For this review, take the finished solid that the model builds, in its own axes (mm). A direction names the side the tool comes from. Coordinates: 2 decimals unless noted, no trailing zeros. Order: outer loops, then holes, each group sorted by start corner. A loop starts at its lowest first (then second) coordinate and runs counter-clockwise, first axis right, second up. Notation, with made-up numbers: M 25.25,-7.75 L 84.25,-7.75 A27 cw 84.25,15.25 Z; hole C 63.5,52 d2. An arc over 180 degrees is marked long. Use CSV: the item, a comma, the result in double quotes.
Autodesk Inventor part; units mm, degrees
ref_plane "Start Plane" through (0, 0, 50.831) normal (0, 0, 1) x (1, 0, 0)
ref_plane "End Plane" through (0, 0, 1320.8) normal (0, 0, 1) x (1, 0, 0)
ref_plane "Work Plane4" through (-2540, 0, 50.831) normal (0, 0, -1) x (-1, 0, 0)
ref_plane "Start Plane" through (0, 0, 50.831) normal (0, 0, 1) x (1, 0, 0)
ref_plane "End Plane" through (0, 0, 1320.8) normal (0, 0, 1) x (1, 0, 0)
sketch "Sketch" plane through (0, 0, 0) normal (0, 0, 1) x (1, 0, 0)
  line L0 (-25.4, -31.75) -> (-25.4, 31.75)
  line L1 (-19.05, 38.1) -> (19.05, 38.1)
  line L2 (25.4, 31.75) -> (25.4, -31.75)
  line L3 (19.05, -38.1) -> (-19.05, -38.1)
  arc A0 (-25.4, -31.75) -> (-19.05, -38.1) centre (-19.05, -31.75) ccw
  arc A1 (-19.05, 38.1) -> (-25.4, 31.75) centre (-19.05, 31.75) ccw
  arc A2 (25.4, 31.75) -> (19.05, 38.1) centre (19.05, 31.75) ccw
  arc A3 (19.05, -38.1) -> (25.4, -31.75) centre (19.05, -31.75) ccw
  arc A4 (-19.05, 34.925) -> (-22.225, 31.75) centre (-19.05, 31.75) ccw
  line L4 (-19.05, 34.925) -> (19.05, 34.925)
  arc A5 (22.225, 31.75) -> (19.05, 34.925) centre (19.05, 31.75) ccw
  line L5 (22.225, 31.75) -> (22.225, -31.75)
  arc A6 (19.05, -34.925) -> (22.225, -31.75) centre (19.05, -31.75) ccw
  line L6 (19.05, -34.925) -> (-19.05, -34.925)
  arc A7 (-22.225, -31.75) -> (-19.05, -34.925) centre (-19.05, -31.75) ccw
  line L7 (-22.225, -31.75) -> (-22.225, 31.75)
  line L8 (0, 55.1812) -> (0, -55.1812) construction
  line L9 (-37.4012, 0) -> (37.4012, 0) construction
  dimension "d10" = 76.2
  dimension "d11" = 50.8
  dimension "d12" = 3.175
  dimension "d15" = 38.1
  dimension "d16" = 25.4
  dimension "d17" = 6.35
extrude "Body" add sketch "Sketch" along normal up to surface (1269.969 mm away) from surface at 50.831
sketch "Sketch3" plane through (0, 0, 0) normal (0, 0, 1) x (1, 0, 0)
  line L0 (0, 0) -> (10, 0)
ref_plane "Work Plane3" through (0, 0, 0) normal (0, -1, 0) x (1, 0, 0)
ref_plane "Work Plane4" through (-2540, 0, 50.831) normal (0, 0, -1) x (-1, 0, 0)
split "Split1" plane through (-2540, 0, 50.831) removes the side toward (0, 0, -1)
sketch "Sketch4" plane through (0, 0, 0) normal (0, -1, 0) x (1, 0, 0)
  line L0 (-2, 50.831) -> (12, 50.831)
  line L1 (-2, 1320.8) -> (12, 1320.8)
  dimension "d19" = 1269.969
equation "\"d10\" = G_H"
equation "\"d11\" = G_W"
equation "\"d12\" = G_T"
equation "\"d15\" = 0.5 * d10"
equation "\"d16\" = 0.5 * d11"
equation "\"d17\" = G_IR"
equation "\"d3\" = G_L"
equation "\"G_W\" = 50.8"
equation "\"G_H\" = 76.2"
equation "\"G_T\" = 3.175"
equation "\"G_IR\" = 6.35"
equation "\"G_L\" = d19"
equation "\"G_OFFSET_START\" = -50.831"
equation "\"G_OFFSET_END\" = 0"
equation "\"d13\" = -G_OFFSET_START"
equation "\"d14\" = G_OFFSET_END + B_L"
equation "\"B_L\" = 1320.8"
properties part number "AISC - 3 x 2 x 1/8 - 49.999" material "Steel, Mild"
Item 1: For faces 5 (the face through (0, -38.1, 677)), 6 (the face through (-22.225, 0, 677)), list the 3-axis set-ups (+Z, -Z, +X, -X, +Y, -Y) from which the entire face can be reached by the end or side of a thin tool; tool diameter is ignored.
Solutions:
face 5,"+Z, -Z, +X, -X, -Y"
face 6,"+Z, -Z"
Item 2: Draft analysis for pull direction X (two halves, no side actions). For faces 1 (the face through (0, -34.925, 677)), 2 (the face through (25.4, 0, 677)), 3 (the face through (22.225, 0, 677)), 4 (the face through (-23, 0, 1320.8)), state which applies: released by +X, released by -X, zero draft, split by the parting line, or undercut.
Solutions:
face 1,"undercut"
face 2,"released by +X"
face 3,"undercut"
face 4,"zero draft"
Item 3: To check wall thickness, follow line 1 along X through (y, z) = (-14.5, 164) (3 decimals); line 2 along Y through (x, z) = (-18, 1145) (3 decimals). State the ranges of each line that lie inside material, in increasing order. Write a range as [from, to].
Solutions:
line 1,"[-25.4, -22.225], [22.225, 25.4]"
line 2,"[-38.1, -34.925], [34.925, 38.1]"
Item 4: Add section C-C on z = 961. State the section outline as (x, y) points (3 decimals).
Solutions:
outline,"M -25.4,-31.75 A6.35 ccw -19.05,-38.1 L 19.05,-38.1 A6.35 ccw 25.4,-31.75 L 25.4,31.75 A6.35 ccw 19.05,38.1 L -19.05,38.1 A6.35 ccw -25.4,31.75 Z; hole M -22.225,-31.75 A3.175 ccw -19.05,-34.925 L 19.05,-34.925 A3.175 ccw 22.225,-31.75 L 22.225,31.75 A3.175 ccw 19.05,34.925 L -19.05,34.925 A3.175 ccw -22.225,31.75 Z"
Item 5: Add section A-A on y = -5. State the section outline as (x, z) points (3 decimals), and give its area (3 significant figures).
Solutions:
outline,"M -25.4,50.831 L -22.225,50.831 L -22.225,1320.8 L -25.4,1320.8 Z; M 22.225,50.831 L 25.4,50.831 L 25.4,1320.8 L 22.225,1320.8 Z"
area,"8,060 mm^2"
Item 6: Add section B-B on x = 7. State the section outline as (y, z) points (3 decimals).
Solutions:
outline,"M -38.1,50.831 L -34.925,50.831 L -34.925,1320.8 L -38.1,1320.8 Z; M 34.925,50.831 L 38.1,50.831 L 38.1,1320.8 L 34.925,1320.8 Z"
